Read the model definition and answer for the solid it produces. Units are mm, in the model's axes. A direction names the side the tool comes from. Give positions to 0.01 mm unless a question says otherwise; leave off trailing zeros. Loops run counter-clockwise (first coordinate to the right, second up) from the corner with the lowest first, then second, coordinate; pieces in that order, holes last. Notation, with made-up numbers: (18.5, -28) - (31.5, -28) arc R29 ccw to (31.5, -3) - close; hole circle Ø11 at (-24, 36). An arc over 180 degrees is marked (long way). Write item = value, one per line.
```python
from build123d import *

# Parameters (mm, degrees)
F0_W     = 101.6
F0_H     = 101.6
F1_DEPTH = 25.4
F3_D     = 24
F3_DEPTH = 12
F3_TIP   = 7.2103274283


with BuildPart() as f1:
    # F0 (on Top) → F1 (new body)
    with BuildSketch(Plane.XY):
        Rectangle(F0_W, F0_H)
    extrude(amount=F1_DEPTH)

    # F3
    with Locations(Plane.XY.offset(25.4)):
        with Locations((-25.4, 25.4), (25.4, 25.4), (0, 0), (25.4, -25.4), (-25.4, -25.4)):
            Hole(F3_D / 2, depth=F3_DEPTH)
            with Locations((0, 0, -(F3_DEPTH + F3_TIP / 2))):  # 118° drill point
                Cone(0, F3_D / 2, F3_TIP, mode=Mode.SUBTRACT)


solid = f1.part
```
1) A cutting plane is placed at B-B on z = 10. Determine the outline of the cut face in (x, y), then the cut area to 3 significant figures.
Output:
outline = (-50.8, -50.8) - (50.8, -50.8) - (50.8, 50.8) - (-50.8, 50.8) - close; hole circle Ø12.68 at (-25.4, -25.4); hole circle Ø12.68 at (-25.4, 25.4); hole circle Ø12.68 at (0, 0); hole circle Ø12.68 at (25.4, -25.4); hole circle Ø12.68 at (25.4, 25.4)
area = 9,690 mm²
2) The mould has two halves that part along Y. Classify faces 3 (the face through (23.75, 24.13, 7.44)), 4 (the face through (-1, 50.8, 13)), 5 (the face through (50.8, -1, 13)): pulls with the +Y half, pulls with the -Y half, needs draft (parallel to the pull), parting line crosses it, or undercut.
Output:
face_3 = undercut
face_4 = pulls with the +Y half
face_5 = needs draft
3) This flat-tipped pin is pushed along its axis until it touches: P1, Ø21.5, axis at x = 25.4, y = -25.4, coming from the +Z side. Where does it stop, or does it pass through?
Output:
P1 = 12.65
4) Find the intervals of material crossed by probe 1 along Y at (x, z) = (25.4, 21.5); probe 2 along X at (y, z) = (-22.5, 19.5), in increasing order.
Output:
probe_1 = -50.8 to -37.4, -13.4 to 13.4, 37.4 to 50.8
probe_2 = -50.8 to -37.04, -13.76 to 13.76, 37.04 to 50.8
5) A tool of negligible diameter and unlimited length cuts with its end or side. For faces 1 (the face through (-1, 1, 0)), 2 (the face through (-22.799, 13.685, 19.316)), from which of +Z, -Z, +X, -X, +Y, -Y can it reach the whole face along a straight path? Write none if from no direction.
Output:
face_1 = -Z, +X, -X, +Y, -Y
face_2 = +Z
6) A cutting plane is placed at A-A on z = 17.5. Determine the outline of the cut face in (x, y), then the cut area to 3 significant figures.
Output:
outline = (-50.8, -50.8) - (50.8, -50.8) - (50.8, 50.8) - (-50.8, 50.8) - close; hole circle Ø24 at (-25.4, -25.4); hole circle Ø24 at (-25.4, 25.4); hole circle Ø24 at (0, 0); hole circle Ø24 at (25.4, -25.4); hole circle Ø24 at (25.4, 25.4)
area = 8,060 mm²
